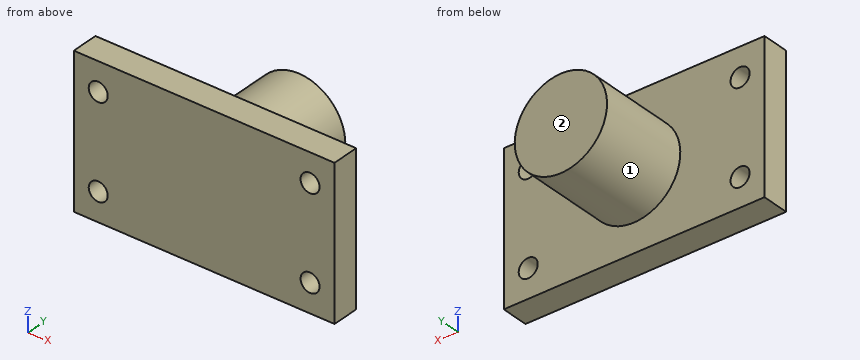
```python
from build123d import *

# Parameters (mm, degrees)
SKETCH_1_W               = 48
SKETCH_1_H               = 27.5
EXTRUDE_1_DEPTH          = 5
SKETCH_2_R               = 8.5
EXTRUDE_2_DEPTH          = 16.87
CUT_EXTRUDE_1_DEPTH      = 60.485686514
CUT_EXTRUDE_1_DEPTH_BACK = 60.485686514
SKETCH_3_R               = 1.75


with BuildPart() as part:
    # 草图1 → 凸台-拉伸1 (new body)
    with BuildSketch(Plane(origin=(0, 0, 0), x_dir=(1, 0, 0), z_dir=(0, 1, 0))):
        with Locations((24, -13.75)):
            Rectangle(SKETCH_1_W, SKETCH_1_H)
    extrude(amount=EXTRUDE_1_DEPTH)

    # 草图2 → 凸台-拉伸2 (add)
    with BuildSketch(Plane(origin=(0, 5, 0), x_dir=(1, 0, 0), z_dir=(0, 1, 0))):
        with Locations(Location((24, -13.75, 0), (0, 0, 270))):
            Circle(SKETCH_2_R)
    extrude(amount=EXTRUDE_2_DEPTH)

    # 草图3 → 切除-拉伸1 (cut, two sides: drawn at the far end of the back side and taken through both)
    with BuildSketch(Plane.XZ.offset(-CUT_EXTRUDE_1_DEPTH_BACK)):
        with Locations(Location((4.5, 22.25, 0), (0, 0, 270))):
            Circle(SKETCH_3_R)
        with Locations(Location((43.5, 22.25, 0), (0, 0, 270))):
            Circle(SKETCH_3_R)
        with Locations(Location((43.5, 5.25, 0), (0, 0, 270))):
            Circle(SKETCH_3_R)
        with Locations(Location((4.5, 5.25, 0), (0, 0, 270))):
            Circle(SKETCH_3_R)
    extrude(amount=CUT_EXTRUDE_1_DEPTH + CUT_EXTRUDE_1_DEPTH_BACK, mode=Mode.SUBTRACT)


solid = part.part
```
Source: CAD feature listing. Evaluate the final solid. Frame: model axes, mm. Face numbers are marked on the shaded views. A direction names the side the tool comes from. Coordinates: 2 decimals unless noted, no trailing zeros. Write each loop counter-clockwise with the first axis right and the second up, starting at its lowest first coordinate (ties: lowest second). Pieces come first, ordered by that corner, then holes. Notation, with made-up numbers: (4, 51) - (55, 51) arc R22 cw to (55, 61) - close; hole circle Ø7 at (73.25, 82). An arc over 180 degrees is marked (long way). Answer as a JSON object with one key per item and string values.
Q1. First-contact query: pin 1 Ø6 at (y, z) = (8.5, 16.5) entering from -X; pin 2 Ø1 at (x, y) = (28, 16.5) entering from -Z; pin 3 Ø8 at (y, z) = (10, 15.5) entering from +X. Flat tips, straight axial feed; report the tip coordinate or a pass-through.
Ans:
{"pin 1": "stops at x = 15.5", "pin 2": "stops at z = 6", "pin 3": "stops at x = 32.5"}
Q2. Section query B-B, the plane z = 4.5. Output: boundary loops of the cut face in (x, y), plus the area to 3 significant figures.
Ans:
{"outline": "(0, 0) - (2.92, 0) - (2.92, 5) - (0, 5) - close; (6.08, 0) - (41.92, 0) - (41.92, 5) - (6.08, 5) - close; (45.08, 0) - (48, 0) - (48, 5) - (45.08, 5) - close", "area": "208 mm2"}
Q3. Section query A-A, the plane x = 43.5. Output: boundary loops of the cut face in (y, z).
Ans:
{"outline": "(0, 0) - (5, 0) - (5, 3.5) - (0, 3.5) - close; (0, 7) - (5, 7) - (5, 20.5) - (0, 20.5) - close; (0, 24) - (5, 24) - (5, 27.5) - (0, 27.5) - close"}
Q4. Set-up query: the marked faces 1 and 2. Return all of +Z, -Z, +X, -X, +Y, -Y with unobstructed straight access to the full face (end or side cutting, diameter ignored); none if empty.
Ans:
{"face 1": "+Y", "face 2": "+Z, -Z, +X, -X, +Y"}
Q5. Section query C-C, the plane y = 2.25. Output: boundary loops of the cut face in (x, z), plus the area to 3 significant figures.
Ans:
{"outline": "(0, 0) - (48, 0) - (48, 27.5) - (0, 27.5) - close; hole circle Ø3.5 at (4.5, 5.25); hole circle Ø3.5 at (4.5, 22.25); hole circle Ø3.5 at (43.5, 5.25); hole circle Ø3.5 at (43.5, 22.25)", "area": "1,280 mm2"}
Q6. Material intervals for line 1 (Z direction, x = 4.5, y = 1.95); line 2 (X direction, y = 3.7, z = 22.25); line 3 (Y direction, x = 19, z = 6.75), sorted ascending. Write a range as [from, to].
Ans:
{"line 1": "z = [0, 3.5], [7, 20.5], [24, 27.5]", "line 2": "x = [0, 2.75], [6.25, 41.75], [45.25, 48]", "line 3": "y = [0, 5]"}
Q7. Section query D-D, the plane z = 13.75. Output: boundary loops of the cut face in (x, y), plus the area to 3 significant figures.
Ans:
{"outline": "(0, 0) - (48, 0) - (48, 5) - (32.5, 5) - (32.5, 21.87) - (15.5, 21.87) - (15.5, 5) - (0, 5) - close", "area": "527 mm2"}
